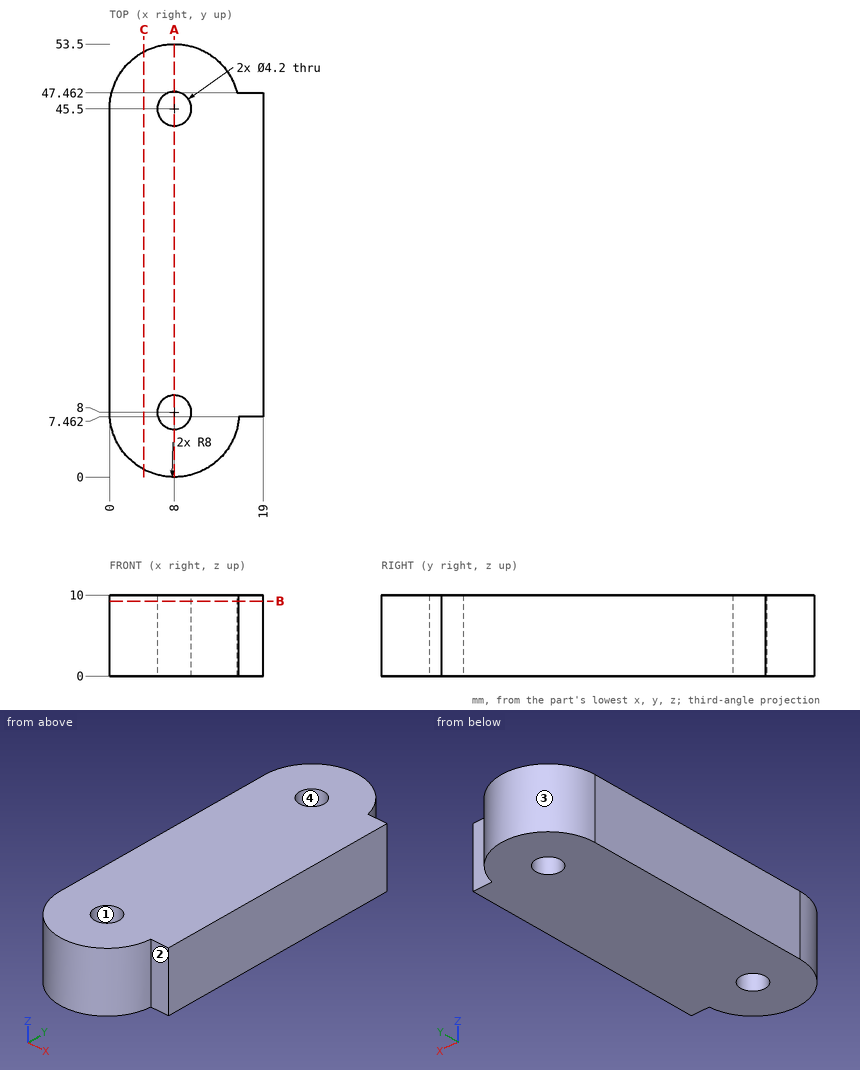
Design review of the part shown in the three views and the two pictorial views. Dimensions are in mm from the part's minimum x, y and z. Give positions to 0.01 mm unless a question says otherwise; leave off trailing zeros. Loops run counter-clockwise (first coordinate to the right, second up) from the corner with the lowest first, then second, coordinate; pieces in that order, holes last. Notation, with made-up numbers: (7.5, 24.5) - (40.5, 24.5) arc R33 ccw to (40.5, 54.5) - close; hole circle Ø10 at (11, -13). An arc over 180 degrees is marked (long way). Answer as a JSON object with one key per item and string values.
Q1. To check wall thickness, follow line 1 along Y through (x, z) = (8, 7.75); line 2 along X through (y, z) = (44.5, 2); line 3 along Y through (x, z) = (5.5, 8.75). State the ranges of each line that lie inside material, in increasing order.
Worked out:
{"line 1": "y = 0 to 5.9, 10.1 to 43.4, 47.6 to 53.5", "line 2": "x = 0 to 6.15, 9.85 to 19", "line 3": "y = 0.4 to 53.1"}
Q2. Add section C-C on x = 4.25. State the section outline as (y, z) points, plus the area to 3 significant figures.
Worked out:
{"outline": "(0.93, 0) - (52.57, 0) - (52.57, 10) - (0.93, 10) - close", "area": "516 mm^2"}
Q3. Mouldability with a two-part tool opening along X and no side actions: class the marked faces 1, 2, 3 and 4 as +X half, -X half, draft (parallel to the pull), parting line (faces both ways), or undercut.
Worked out:
{"face 1": "undercut", "face 2": "draft", "face 3": "parting line", "face 4": "undercut"}
Q4. Add section B-B on z = 9.25. State the section outline as (x, y) points, plus the area to 3 significant figures.
Worked out:
{"outline": "(0, 8) arc R8 ccw to (15.98, 7.46) - (19, 7.46) - (19, 47.46) - (15.76, 47.46) arc R8 ccw to (0, 45.5) - close; hole circle Ø4.2 at (8, 8); hole circle Ø4.2 at (8, 45.5)", "area": "894 mm^2"}
Q5. Insertion check: pin 1 (3 mm diameter, centred on x = 12, z = 1.5, fed in from -Y); pin 2 (1 mm diameter, centred on x = 18, z = 3, fed in from +Y); pin 3 (1.5 mm diameter, centred on x = 18, z = 3.5, fed in from -Y). Each pin has a flat end and moves straight along its axis. Give the tip position at first contact, or say it passes through.
Worked out:
{"pin 1": "stops at y = 0.4", "pin 2": "stops at y = 47.46", "pin 3": "stops at y = 7.46"}
Q6. Add section A-A on x = 8. State the section outline as (y, z) points, plus the area to 3 significant figures.
Worked out:
{"outline": "(0, 0) - (5.9, 0) - (5.9, 10) - (0, 10) - close; (10.1, 0) - (43.4, 0) - (43.4, 10) - (10.1, 10) - close; (47.6, 0) - (53.5, 0) - (53.5, 10) - (47.6, 10) - close", "area": "451 mm^2"}
